Verification items for the finished model (mm, model axes). Round coordinates to 2 decimals unless told otherwise and drop trailing zeros. Write each loop counter-clockwise with the first axis right and the second up, starting at its lowest first coordinate (ties: lowest second). Pieces come first, ordered by that corner, then holes. Notation, with made-up numbers: (18, -12.75) -> (28, -12.75) arc R24 ccw to (28, 4.25) -> close; hole circle Ø3 at (80, 47.25). An arc over 180 degrees is marked (long way). Answer as a JSON object with one key per item and string values. Group by question number.
(1) Sectioned sample at A-A on x = -1. Record the cut outline in (y, z).
(2) Gauge pin test, flat ends, axial feed: pin 1 Ø2.5 at (y, z) = (89, 2) entering from -X; pin 2 Ø2.5 at (x, z) = (-47, 3.5) entering from +Y; pin 3 Ø1.4 at (y, z) = (98.5, 1.5) entering from -X. Record the tip position at first contact, or that the pin passes through.
(3) Sectioned sample at B-B on y = 43.5. Record the cut outline in (x, z), and give its area (3 significant figures).
(4) Scan lines: L1, parallel to Y at x = 25.5, z = 2.05; L2, parallel to X at y = 53, z = 4.35. Record each from-to range of solid material in increasing order. Write a range as from..to.
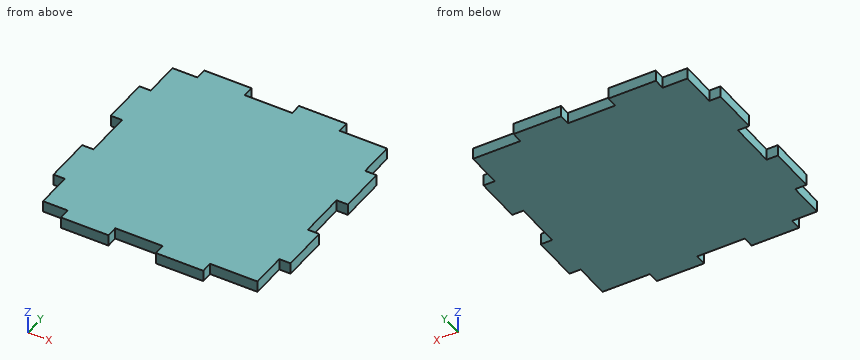
```python
from build123d import *

# Parameters (mm, degrees)
SKETCH2_W           = 100
SKETCH2_H           = 100
BOSS_EXTRUDE1_DEPTH = 4.7625
CAVITY1_START       = -50
CAVITY1_OUTLINE_W   = 20
CAVITY1_OUTLINE_H   = 4.7625
CAVITY1_DEPTH       = 4.7625
CAVITY1_START_2     = 45.2375
CAVITY1_2_OUTLINE_W = 20
CAVITY1_2_OUTLINE_H = 4.7625
CAVITY1_2_DEPTH     = 4.7625
CAVITY1_START_3     = -14.7625
CAVITY1_3_OUTLINE_W = 4.7625
CAVITY1_3_OUTLINE_H = 4.7625
CAVITY1_3_DEPTH     = 20
CAVITY1_START_4     = 25.2375
CAVITY1_4_OUTLINE_W = 4.7625
CAVITY1_4_OUTLINE_H = 4.7625
CAVITY1_4_DEPTH     = 20
CAVITY1_START_5     = -45.2375
CAVITY1_5_OUTLINE_W = 4.7625
CAVITY1_5_OUTLINE_H = 4.7625
CAVITY1_5_DEPTH     = 10.475


# Read off the part's stored shape, not the designer's step: Cavity1
with BuildPart() as part:
    # Sketch2 → Boss-Extrude1 (new body)
    with BuildSketch(Plane.XY.offset(4.7625)):
        with Locations((0, 50)):
            Rectangle(SKETCH2_W, SKETCH2_H)
    extrude(amount=-BOSS_EXTRUDE1_DEPTH)

    # Cavity1 outline → Cavity1 (cut)
    with BuildSketch(Plane.YZ.offset(CAVITY1_START)):
        with Locations((10, 2.38125)):
            Rectangle(CAVITY1_OUTLINE_W, CAVITY1_OUTLINE_H)
        with Locations((50, 2.38125)):
            Rectangle(CAVITY1_OUTLINE_W, CAVITY1_OUTLINE_H)
        with Locations((90, 2.38125)):
            Rectangle(CAVITY1_OUTLINE_W, CAVITY1_OUTLINE_H)
    extrude(amount=CAVITY1_DEPTH, mode=Mode.SUBTRACT)

    # Cavity1 2 outline → Cavity1 2 (cut)
    with BuildSketch(Plane.YZ.offset(CAVITY1_START_2)):
        with Locations((10, 2.38125)):
            Rectangle(CAVITY1_2_OUTLINE_W, CAVITY1_2_OUTLINE_H)
        with Locations((50, 2.38125)):
            Rectangle(CAVITY1_2_OUTLINE_W, CAVITY1_2_OUTLINE_H)
        with Locations((90, 2.38125)):
            Rectangle(CAVITY1_2_OUTLINE_W, CAVITY1_2_OUTLINE_H)
    extrude(amount=CAVITY1_2_DEPTH, mode=Mode.SUBTRACT)

    # Cavity1 3 outline → Cavity1 3 (cut)
    with BuildSketch(Plane.YZ.offset(CAVITY1_START_3)):
        with Locations((2.38125, 2.38125)):
            Rectangle(CAVITY1_3_OUTLINE_W, CAVITY1_3_OUTLINE_H)
        with Locations((97.61875, 2.38125)):
            Rectangle(CAVITY1_3_OUTLINE_W, CAVITY1_3_OUTLINE_H)
    extrude(amount=CAVITY1_3_DEPTH, mode=Mode.SUBTRACT)

    # Cavity1 4 outline → Cavity1 4 (cut)
    with BuildSketch(Plane.YZ.offset(CAVITY1_START_4)):
        with Locations((2.38125, 2.38125)):
            Rectangle(CAVITY1_4_OUTLINE_W, CAVITY1_4_OUTLINE_H)
        with Locations((97.61875, 2.38125)):
            Rectangle(CAVITY1_4_OUTLINE_W, CAVITY1_4_OUTLINE_H)
    extrude(amount=CAVITY1_4_DEPTH, mode=Mode.SUBTRACT)

    # Cavity1 5 outline → Cavity1 5 (cut)
    with BuildSketch(Plane.YZ.offset(CAVITY1_START_5)):
        with Locations((2.38125, 2.38125)):
            Rectangle(CAVITY1_5_OUTLINE_W, CAVITY1_5_OUTLINE_H)
        with Locations((97.61875, 2.38125)):
            Rectangle(CAVITY1_5_OUTLINE_W, CAVITY1_5_OUTLINE_H)
    extrude(amount=CAVITY1_5_DEPTH, mode=Mode.SUBTRACT)


solid = part.part
```
Computed values:
{
 "1": {"outline": "(4.76, 0) -> (95.24, 0) -> (95.24, 4.76) -> (4.76, 4.76) -> close"},
 "2": {"pin 1": "x = -45.24", "pin 2": "y = 80", "pin 3": "x = -34.76"},
 "3": {"outline": "(-45.24, 0) -> (45.24, 0) -> (45.24, 4.76) -> (-45.24, 4.76) -> close", "area": "431 mm2"},
 "4": {"L1": "4.76..95.24", "L2": "-45.24..45.24"}
}
